Here's how the part is built. I have some questions about the finished solid (model axes, mm). A direction names the side the tool comes from. Coordinates: 2 decimals unless noted, no trailing zeros. Write each loop counter-clockwise with the first axis right and the second up, starting at its lowest first coordinate (ties: lowest second). Pieces come first, ordered by that corner, then holes.
```python
from build123d import *

# Parameters (mm, degrees)
BOSS_EXTRUDE1_DEPTH = 8.5
CUT_EXTRUDE2_START  = -2.5
SKETCH2_W           = 17.5
SKETCH2_H           = 13.4
CUT_EXTRUDE2_DEPTH  = 28.033878851
CUT_EXTRUDE3_DEPTH  = 17
CUT_EXTRUDE4_DEPTH  = 17
SKETCH5_W           = 1.8
SKETCH5_H           = 3.5
BOSS_EXTRUDE2_DEPTH = 1.5
SKETCH6_W           = 3.5
SKETCH6_H           = 1.8
BOSS_EXTRUDE3_DEPTH = 1.5


with BuildPart() as part:
    # Sketch1 → Boss-Extrude1 (new, symmetric)
    with BuildSketch(Plane.XY):
        Polygon((0, 20), (2.5, 20), (20, 2.5), (20, 0), (0, 0), align=None)
    extrude(amount=BOSS_EXTRUDE1_DEPTH, both=True)

    # Sketch2 → Cut-Extrude2 (cut, through all)
    with BuildSketch(Plane.XZ.offset(CUT_EXTRUDE2_START)):
        with Locations((11.25, 0)):
            Rectangle(SKETCH2_W, SKETCH2_H)
    extrude(amount=-CUT_EXTRUDE2_DEPTH, mode=Mode.SUBTRACT)

    # Sketch3 → Cut-Extrude3 (cut)
    with BuildSketch(Plane(origin=(0, 2.5, 0), x_dir=(1, 0, 0), z_dir=(0, 1, 0))):
        with BuildLine():
            Line((8.25, 3), (11.75, 3))
            ThreePointArc((11.75, 3), (14.75, 0), (11.75, -3))
            Line((11.75, -3), (8.25, -3))
            ThreePointArc((8.25, -3), (5.25, 0), (8.25, 3))
        make_face()
    extrude(amount=-CUT_EXTRUDE3_DEPTH, mode=Mode.SUBTRACT)

    # Sketch4 → Cut-Extrude4 (cut)
    with BuildSketch(Plane(origin=(2.5, 0, 0), x_dir=(0, 0, -1), z_dir=(1, 0, 0))):
        with BuildLine():
            Line((-3, 8.25), (-3, 11.75))
            ThreePointArc((-3, 11.75), (0, 14.75), (3, 11.75))
            Line((3, 11.75), (3, 8.25))
            ThreePointArc((3, 8.25), (0, 5.25), (-3, 8.25))
        make_face()
    extrude(amount=-CUT_EXTRUDE4_DEPTH, mode=Mode.SUBTRACT)

    # Sketch5 → Boss-Extrude2 (add)
    with BuildSketch(Plane.XZ):
        with Locations((2, 0)):
            Rectangle(SKETCH5_W, SKETCH5_H)
        with Locations((18, 0)):
            Rectangle(SKETCH5_W, SKETCH5_H)
    extrude(amount=BOSS_EXTRUDE2_DEPTH)

    # Sketch6 → Boss-Extrude3 (add)
    with BuildSketch(Plane.ZY):
        with Locations((0, 2)):
            Rectangle(SKETCH6_W, SKETCH6_H)
        with Locations((0, 18)):
            Rectangle(SKETCH6_W, SKETCH6_H)
    extrude(amount=BOSS_EXTRUDE3_DEPTH)


solid = part.part
```
1) Imagine slicing it at D-D on y = 18. Please give me the cut outline in (x, z).
Values follow:
outline: (-1.5, -1.75) - (0, -1.75) - (0, -8.5) - (4.5, -8.5) - (4.5, -6.7) - (2.5, -6.7) - (2.5, 6.7) - (4.5, 6.7) - (4.5, 8.5) - (0, 8.5) - (0, 1.75) - (-1.5, 1.75) - close
2) Imagine slicing it at C-C on x = 2. Please give me the cut outline in (y, z), then the cut area to 3 significant figures.
Values follow:
outline: (-1.5, -1.75) - (0, -1.75) - (0, -8.5) - (20, -8.5) - (20, 8.5) - (0, 8.5) - (0, 1.75) - (-1.5, 1.75) - close; hole (8.25, -3) - (11.75, -3) arc R3 ccw to (11.75, 3) - (8.25, 3) arc R3 ccw to start
area: 296 mm2
3) On a 3-axis mill with a long thin cutter (end or side, diameter ignored), from which of +Z, -Z, +X, -X, +Y, -Y can I reach the whole of each face in a straight line? I mean faces 1 (the face through (10, 1, -3)), 2 (the face through (-1, 18.9, 0)), 3 (the face through (-1, 17.1, 0)), 4 (the face through (2, -1, 1.75)), 5 (the face through (1, 10, -3)). Say none if no direction works.
Values follow:
face 1: +Y, -Y
face 2: +Z, -Z, -X, +Y
face 3: +Z, -Z, -X
face 4: +Z, +X, -X, -Y
face 5: +X, -X
4) We'd pull the mould along X, two halves only. Please class faces 6 (the face through (-1.5, 2, 0)), 7 (the face through (-1, 2.9, 0)), 8 (the face through (17.1, -1, 0)): pulls with the +X half, pulls with the -X half, needs draft (parallel to the pull), parting line crosses it, or undercut.
Values follow:
face 6: pulls with the -X half
face 7: needs draft
face 8: undercut
5) Imagine slicing it at B-B on y = 10.5. Please give me the cut outline in (x, z), then the cut area to 3 significant figures.
Values follow:
outline: (0, -8.5) - (12, -8.5) - (12, -6.7) - (2.5, -6.7) - (2.5, -3) - (0, -3) - close; (0, 3) - (2.5, 3) - (2.5, 6.7) - (12, 6.7) - (12, 8.5) - (0, 8.5) - close
area: 61.7 mm2
6) Imagine slicing it at A-A on z = 0. Count the separate pieces of the cut face and the enclosed holes in it, then the cut area to 4 significant figures.
Values follow:
separate pieces: 3
enclosed holes: 0
area: 57.05 mm2
7) I need wall thicknesses on probe 1 along Y at (x, z) = (0.5, 0); probe 2 along Z at (x, y) = (4.75, 3.75); probe 3 along Z at (x, y) = (0.25, 11). Which ranges of each line are inside material? Lowest first, please.
Values follow:
probe 1: y = 0 to 5.25, 14.75 to 20
probe 2: z = -8.5 to -6.7, 6.7 to 8.5
probe 3: z = -8.5 to -3, 3 to 8.5
8) Will these pins go through, and if not, where does the flat tip stop? pin 1 (1.2 mm diameter, centred on x = -1, z = -1, fed in from -Y); pin 2 (1.6 mm diameter, centred on x = 1.5, y = -1, fed in from +Z); pin 3 (4 mm diameter, centred on x = 9, z = 2, fed in from -Y).
Values follow:
pin 1: stops at y = 1.1
pin 2: stops at z = 1.75
pin 3: stops at y = 0
